from build123d import *

# Parameters (mm, degrees)
CORTE_EXTRUS_O1_START = -0.5
ESBO_O2_W             = 9.2
ESBO_O2_H             = 1
CORTE_EXTRUS_O1_DEPTH = 10


with BuildPart() as part:
    # Esboço1 → Revolução1 (revolve)
    with BuildSketch(Plane(origin=(0, 0, 0), x_dir=(1, 0, 0), z_dir=(0, 1, 0))):
        with BuildLine():
            Line((1.9, 0), (4, 0))
            add(Edge.make_bspline(
                [(4, 0), (4, 1.5), (0, 1.5)],
                knots=[0, 0, 0, 1.570796327, 1.570796327, 1.570796327], degree=2, weights=[1, 0.707106781, 1]))
            Line((0, 1.5), (0, 0))
            Line((0, 0), (0, -35))
            Line((0, -35), (1.9, -35))
            Line((1.9, -35), (1.9, 0))
        make_face()
    revolve(axis=Axis((0, 0, 0), (0, 0, 1)))

    # Esboço2 → Corte-extrusão1 (cut)
    with BuildSketch(Plane.XY.offset(CORTE_EXTRUS_O1_START)):
        Rectangle(ESBO_O2_W, ESBO_O2_H)
    extrude(amount=-CORTE_EXTRUS_O1_DEPTH, mode=Mode.SUBTRACT)


solid = part.part
For this review, take the finished solid that the model builds, in its own axes (mm). A direction names the side the tool comes from. Coordinates: 2 decimals unless noted, no trailing zeros. Order: outer loops, then holes, each group sorted by start corner. A loop starts at its lowest first (then second) coordinate and runs counter-clockwise, first axis right, second up. Notation, with made-up numbers: (56.25, 36) -> (66.25, 36) arc R19 ccw to (66.25, 69) -> close; hole circle Ø10 at (-31, 72.25). An arc over 180 degrees is marked (long way). Return JSON: item names as keys, results as strings.
1. The part is to be moulded in two halves that separate along Y. For faces 1 (the cylindrical face through (-1.9, 0.08, 17.26)), 2 (the flat face through (-2, -1, 0)), 3 (the flat face through (0, 0, -0.5)), say which applies: +Y half, -Y half, draft (parallel to the pull), parting line (faces both ways), or undercut.
Answer block:
{"face 1": "parting line", "face 2": "draft", "face 3": "undercut"}
2. Machinability: for faces 4 (the flat face through (0, 0, 35)), 5 (the flat face through (0, -0.5, -1)), which of the approach directions +Z, -Z, +X, -X, +Y, -Y give a long, thin tool a straight path to every point of the face, cutting with its end or side? Answer none if there is none.
Answer block:
{"face 4": "+Z, +X, -X, +Y, -Y", "face 5": "-Z, +X, -X"}
3. We need section A-A on z = 7.5. Write out the cut boundary in (x, y), and give its area (3 significant figures).
Answer block:
{"outline": "circle Ø3.8 at (0, 0)", "area": "11.3 mm²"}
4. For pin 1 Ø4 at (x, z) = (3, 22.5) entering from -Y; pin 2 Ø3 at (x, z) = (3, 30) entering from -Y; pin 3 Ø0.8 at (x, y) = (1.5, 0) entering from -Z, all flat-tipped, find the tip position at first contact; note any pin that passes through.
Answer block:
{"pin 1": "y = -1.62", "pin 2": "y = -1.17", "pin 3": "z = -0.5"}
5. For line 1 (Z direction, x = -1.25, y = 0); line 2 (Y direction, x = 0.25, z = 6); line 3 (Z direction, x = -0.25, y = -1), list the stretches that pass through material, from the lowest coordinate up. Write a range as from..to.
Answer block:
{"line 1": "-0.5..35", "line 2": "-1.88..1.88", "line 3": "-1.45..35"}
